Here's how the part is built. I have some questions about the finished solid (model axes, mm). A direction names the side the tool comes from. Coordinates: 2 decimals unless noted, no trailing zeros. Order: outer loops, then holes, each group sorted by start corner. A loop starts at its lowest first (then second) coordinate and runs counter-clockwise, first axis right, second up.
```python
from build123d import *

# Parameters (mm, degrees)
EXTRUDE_1_DEPTH     = 14.8
EXTRUDE_2_DEPTH     = 13.8
CUT_EXTRUDE_1_DEPTH = 12
FILLET_1_R          = 0.7
SKETCH_4_R          = 4.382397862
CUT_EXTRUDE_2_DEPTH = 1


with BuildPart() as part:
    # ｽｹｯﾁ1 → ﾎﾞｽ - 押し出し1 (new body)
    with BuildSketch(Plane.XY):
        Polygon((0, 0), (8.3, -0.120571415), (8.3, 13.279428585), (6.6, 13.279428585), (6.6, 20.279428585), (4.9, 20.279428585), (4.9, 21.63120639), (-4.9, 21.63120639), (-4.9, 20.279428585), (-6.6, 20.279428585), (-6.6, 13.279428585), (-8.3, 13.279428585), (-8.3, -0.120571415), align=None)
    extrude(amount=EXTRUDE_1_DEPTH)

    # ｽｹｯﾁ2 → ﾎﾞｽ - 押し出し2 (add)
    with BuildSketch(Plane.XY.offset(14.8)):
        Polygon((-6.3, 1.908692951), (0, 2.000211013), (6.3, 1.908692951), (6.3, 11.279428585), (4.6, 11.279428585), (4.6, 18.279428585), (2.9, 18.279428585), (2.9, 19.63120639), (-2.9, 19.63120639), (-2.9, 18.279428585), (-4.6, 18.279428585), (-4.6, 11.279428585), (-6.3, 11.279428585), align=None)
    extrude(amount=EXTRUDE_2_DEPTH)

    # ｽｹｯﾁ3 → ｶｯﾄ - 押し出し1 (cut)
    with BuildSketch(Plane(origin=(0, 0, 0), x_dir=(-1, 0, 0), z_dir=(0, 0, -1))):
        Polygon((0, 1.000105507), (7.3, 0.894060768), (7.3, 12.279428585), (5.6, 12.279428585), (5.6, 19.279428585), (3.9, 19.279428585), (3.9, 20.63120639), (-3.9, 20.63120639), (-3.9, 19.279428585), (-5.6, 19.279428585), (-5.6, 12.279428585), (-7.3, 12.279428585), (-7.3, 0.894060768), align=None)
    extrude(amount=-CUT_EXTRUDE_1_DEPTH, mode=Mode.SUBTRACT)

    # ﾌｨﾚｯﾄ1
    fillet_1_edges = [part.edges().sort_by_distance(p)[0] for p in [
        (-8.3, 13.279428585, 7.4),
        (-6.6, 20.279428585, 7.4),
        (-4.9, 21.63120639, 7.4),
        (4.9, 21.63120639, 7.4),
        (6.6, 20.279428585, 7.4),
        (8.3, 13.279428585, 7.4),
        (8.3, -0.120571415, 7.4),
        (-6.3, 11.279428585, 21.7),
        (-6.3, 1.908692951, 21.7),
        (6.3, 1.908692951, 21.7),
        (6.3, 11.279428585, 21.7),
        (4.6, 18.279428585, 21.7),
        (2.9, 19.63120639, 21.7),
        (-2.9, 19.63120639, 21.7),
        (-4.6, 18.279428585, 21.7),
    ]]
    fillet(fillet_1_edges, radius=FILLET_1_R)

    # ｽｹｯﾁ4 → ｶｯﾄ - 押し出し2 (cut)
    with BuildSketch(Plane.XY.offset(28.6)):
        with Locations((0, 10.579428585)):
            Circle(SKETCH_4_R)
    extrude(amount=-CUT_EXTRUDE_2_DEPTH, mode=Mode.SUBTRACT)


solid = part.part
```
Q1. We'd pull the mould along X, two halves only. Please class faces 1 (the flat face through (-3, 7, 28.6)), 2 (the flat face through (-6.6, 16, 7)), 3 (the flat face through (5, 19.279, 6)), 4 (the flat face through (-5.6, 16, 6)): pulls with the +X half, pulls with the -X half, needs draft (parallel to the pull), parting line crosses it, or undercut.
Q2. For faces 5 (the flat face through (-7.3, 7, 6)), 6 (the flat face through (-7, 13.279, 7)), 7 (the flat face through (-4.6, 14, 22)), which set-ups out of +Z, -Z, +X, -X, +Y, -Y let a thin tool reach every point of the face, with its end or its side?
Q3. If we section it at D-D on z = 19.25: Write out the boundary of the cut face in (x, y).
Q4. I need wall thicknesses on L1, parallel to Y at x = 0.5, z = 8.25; L2, parallel to X at y = 2.75, z = 1.5; L3, parallel to X at y = 17.25, z = 3.75. Which ranges of each line are inside material? Lowest first, please.
Q5. Will these pins go through, and if not, where does the flat tip stop? pin 1 (12 mm diameter, centred on y = 7.5, z = 24.5, fed in from +X); pin 2 (1.5 mm diameter, centred on x = -6, z = 23, fed in from -Y); pin 3 (0.5 mm diameter, centred on x = -5, z = 4, fed in from -Y).
Q6. If we section it at B-B on x = -1.25: Write out the boundary of the cut face in (y, z), then the cut area to 3 significant figures.
Q7. If we section it at C-C on y = 14.25: Write out the boundary of the cut face in (x, z).
Reply:
1. face 1: needs draft
1. face 2: pulls with the -X half
1. face 3: undercut
1. face 4: undercut
2. face 5: -Z
2. face 6: +Z, -Z, -X, +Y
2. face 7: +Z, -X, +Y
3. outline: (-6.3, 2.62) arc R0.7 ccw to (-5.59, 1.92) - (0, 2) - (5.59, 1.92) arc R0.7 ccw to (6.3, 2.62) - (6.3, 10.58) arc R0.7 ccw to (5.6, 11.28) - (4.6, 11.28) - (4.6, 17.58) arc R0.7 ccw to (3.9, 18.28) - (2.9, 18.28) - (2.9, 18.93) arc R0.7 ccw to (2.2, 19.63) - (-2.2, 19.63) arc R0.7 ccw to (-2.9, 18.93) - (-2.9, 18.28) - (-3.9, 18.28) arc R0.7 ccw to (-4.6, 17.58) - (-4.6, 11.28) - (-5.6, 11.28) arc R0.7 ccw to (-6.3, 10.58) - close
4. L1: y = -0.01 to 0.99, 20.63 to 21.63
4. L2: x = -8.3 to -7.3, 7.3 to 8.3
4. L3: x = -6.6 to -5.6, 5.6 to 6.6
5. pin 1: stops at x = 6.3
5. pin 2: stops at y = 1.92
5. pin 3: stops at y = -0.08
6. outline: (-0.02, 0) - (0.98, 0) - (0.98, 12) - (20.63, 12) - (20.63, 0) - (21.63, 0) - (21.63, 14.8) - (19.63, 14.8) - (19.63, 28.6) - (14.78, 28.6) - (14.78, 27.6) - (6.38, 27.6) - (6.38, 28.6) - (1.98, 28.6) - (1.98, 14.8) - (-0.02, 14.8) - close
6. area: 320 mm2
7. outline: (-6.6, 0) - (-5.6, 0) - (-5.6, 12) - (5.6, 12) - (5.6, 0) - (6.6, 0) - (6.6, 14.8) - (4.6, 14.8) - (4.6, 28.6) - (2.39, 28.6) - (2.39, 27.6) - (-2.39, 27.6) - (-2.39, 28.6) - (-4.6, 28.6) - (-4.6, 14.8) - (-6.6, 14.8) - close
